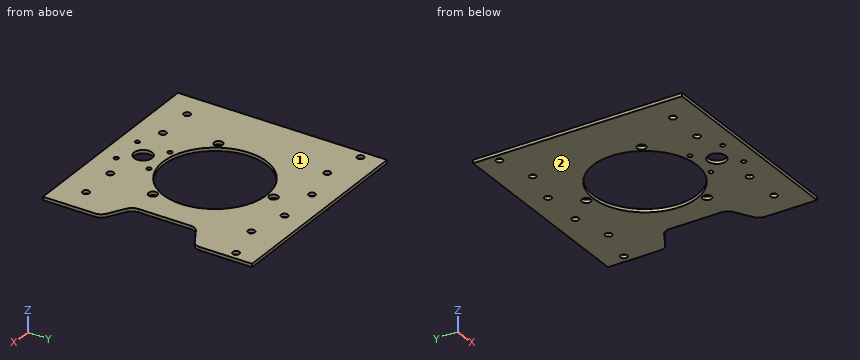
```python
from build123d import *

# Parameters (mm, degrees)
SKETCH1_W               = 203.2
SKETCH1_H               = 203.2
BOSS_EXTRUDE1_DEPTH     = 3.175
SKETCH8_R               = 50.5
SKETCH8_R_2             = 4.25
CUT_EXTRUDE3_DEPTH      = 144.719172782
CUT_EXTRUDE4_DEPTH      = 144.719172782
F_1_4_CLEARANCE_HOLE2_D = 6.5278
F_1_4_CLEARANCE_HOLE1_D = 6.5278
F_8_CLEARANCE_HOLE2_D   = 4.3053
SKETCH19_R              = 8.73125
CUT_EXTRUDE5_DEPTH      = 144.719172782


with BuildPart() as part:
    # Sketch1 → Boss-Extrude1 (new body)
    with BuildSketch(Plane.XY):
        Rectangle(SKETCH1_W, SKETCH1_H)
    extrude(amount=-BOSS_EXTRUDE1_DEPTH)

    # Sketch8 → Cut-Extrude3 (cut, through all)
    with BuildSketch(Plane.XY):
        Circle(SKETCH8_R)
        with Locations((0, 57)):
            Circle(SKETCH8_R_2)
        with Locations((-49.363448016, -28.5)):
            Circle(SKETCH8_R_2)
        with Locations((49.363448016, -28.5)):
            Circle(SKETCH8_R_2)
    extrude(amount=-CUT_EXTRUDE3_DEPTH, mode=Mode.SUBTRACT)

    # Sketch10 → Cut-Extrude4 (cut, through all)
    with BuildSketch(Plane.XY):
        with BuildLine():
            Line((96.8375, 42.814327494), (80.9625, 33.648891971))
            ThreePointArc((80.9625, 33.648891971), (77.476108029, 30.1625), (76.2, 25.4))
            Line((76.2, 25.4), (76.2, -25.4))
            ThreePointArc((76.2, -25.4), (77.476108029, -30.1625), (80.9625, -33.648891971))
            Line((80.9625, -33.648891971), (96.8375, -42.814327494))
            ThreePointArc((96.8375, -42.814327494), (100.323891971, -46.300719465), (101.6, -51.063219465))
            Line((101.6, -51.063219465), (101.6, 51.063219465))
            ThreePointArc((101.6, 51.063219465), (100.323891971, 46.300719465), (96.8375, 42.814327494))
        make_face()
    extrude(amount=-CUT_EXTRUDE4_DEPTH, mode=Mode.SUBTRACT)

    # 1/4 Clearance Hole2 (through all)
    with Locations(Plane.XY):
        with Locations((76.2, -76.2), (39.553111932, -76.2), (-39.553111932, -76.2), (-76.2, -76.2)):
            Hole(F_1_4_CLEARANCE_HOLE2_D / 2)

    # 1/4 Clearance Hole1 (through all)
    with Locations(Plane.XY):
        with Locations((-93.6625, 80.9625), (-57.15, 72.23125), (-20.6375, 80.9625), (20.6375, 80.9625), (57.15, 72.23125), (93.6625, 80.9625)):
            Hole(F_1_4_CLEARANCE_HOLE1_D / 2)

    # #8 Clearance Hole2 (through all)
    with Locations(Plane.XY):
        with Locations((-15.874990337, -53.95749371), (15.874990337, -53.95749371), (-15.874990337, -85.74250629), (15.874990337, -85.74250629)):
            Hole(F_8_CLEARANCE_HOLE2_D / 2)

    # Sketch19 → Cut-Extrude5 (cut, through all)
    with BuildSketch(Plane.XY):
        with Locations((0, -69.85)):
            Circle(SKETCH19_R)
    extrude(amount=-CUT_EXTRUDE5_DEPTH, mode=Mode.SUBTRACT)


solid = part.part
```
The model under review builds one solid part; all positions refer to its coordinate system, in mm. Face numbers are marked on the shaded views. Round coordinates to 2 decimals unless told otherwise and drop trailing zeros. Loops run counter-clockwise (first coordinate to the right, second up) from the corner with the lowest first, then second, coordinate; pieces in that order, holes last. Notation, with made-up numbers: M 36.5,-26.75 L 77.5,-26.75 A20 ccw 77.5,9.25 Z; hole C 6,69.5 d10. An arc over 180 degrees is marked long. Put each result on its own line as item: value.
Q1. For pin 1 (7.5 mm diameter, centred on x = 0, y = 57, fed in from +Z), flat-tipped, find the tip position at first contact; note if it passes through.
Result set:
pin 1: passes through
Q2. Consider section D-D, the plane y = -28.5. Give the boundary of the cut face in (x, z) (3 decimals).
Result set:
outline: M -101.6,-3.175 L -53.613,-3.175 L -53.613,0 L -101.6,0 Z; M -45.113,-3.175 L -41.689,-3.175 L -41.689,0 L -45.113,0 Z; M 41.689,-3.175 L 45.113,-3.175 L 45.113,0 L 41.689,0 Z; M 53.613,-3.175 L 76.719,-3.175 L 76.719,0 L 53.613,0 Z
Q3. Consider section C-C, the plane x = 0. Give the boundary of the cut face in (y, z) (3 decimals).
Result set:
outline: M -101.6,-3.175 L -78.581,-3.175 L -78.581,0 L -101.6,0 Z; M -61.119,-3.175 L -50.5,-3.175 L -50.5,0 L -61.119,0 Z; M 50.5,-3.175 L 52.75,-3.175 L 52.75,0 L 50.5,0 Z; M 61.25,-3.175 L 101.6,-3.175 L 101.6,0 L 61.25,0 Z
Q4. Consider section A-A, the plane x = 57.15. Give the boundary of the cut face in (y, z) (3 decimals).
Result set:
outline: M -101.6,-3.175 L 68.967,-3.175 L 68.967,0 L -101.6,0 Z; M 75.495,-3.175 L 101.6,-3.175 L 101.6,0 L 75.495,0 Z
Q5. Consider section B-B, the plane y = 0. Give the boundary of the cut face in (x, z) (3 decimals).
Result set:
outline: M -101.6,-3.175 L -50.5,-3.175 L -50.5,0 L -101.6,0 Z; M 50.5,-3.175 L 76.2,-3.175 L 76.2,0 L 50.5,0 Z
Q6. Mouldability with a two-part tool opening along Z and no side actions: class the marked faces 1 and 2 as released by +Z, released by -Z, zero draft, split by the parting line, or undercut.
Result set:
face 1: released by +Z
face 2: released by -Z
Q7. To check wall thickness, follow L1, parallel to X at y = 71.5, z = -2.65; L2, parallel to X at y = 83.5, z = -2.2; L3, parallel to Y at x = -41.5, z = -1.4. State the ranges of each line that lie inside material, in increasing order.
Result set:
L1: x = -101.6 to -60.33, -53.97 to 53.97, 60.33 to 101.6
L2: x = -101.6 to -95.72, -91.61 to -22.69, -18.58 to 18.58, 22.69 to 91.61, 95.72 to 101.6
L3: y = -101.6 to -78.82, -73.58 to -28.77, 28.77 to 101.6
